from build123d import *

# Parameters (mm, degrees)
SKETCH1_R           = 5.85
SKETCH1_W           = 22.669
SKETCH1_H           = 11.7
BOSS_EXTRUDE1_DEPTH = 5.6


with BuildPart() as part:
    # Sketch1 → Boss-Extrude1 (new body)
    with BuildSketch(Plane.XY):
        Polygon((702.290264671, 402.743983564), (702.290264671, 391.585983564), (697.040264671, 391.585983564), (697.040264671, 387.985983564), (748.040264671, 387.985983564), (748.040264671, 393.985983564), (742.790264671, 393.985983564), (742.790264671, 400.343983564), (748.040264671, 400.343983564), (748.040264671, 406.343983564), (697.040264671, 406.343983564), (697.040264671, 402.743983564), align=None)
        with Locations((709.880764671, 397.164983564)):
            Circle(SKETCH1_R, mode=Mode.SUBTRACT)
        with Locations((728.805764671, 397.164983564)):
            Rectangle(SKETCH1_W, SKETCH1_H, mode=Mode.SUBTRACT)
    extrude(amount=BOSS_EXTRUDE1_DEPTH)


solid = part.part
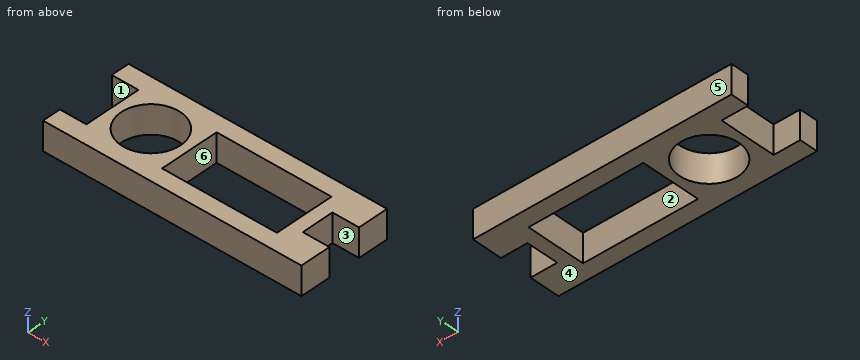
Read the model definition and answer for the solid it produces. Units are mm, in the model's axes. Face numbers are marked on the shaded views. A direction names the side the tool comes from. Round coordinates to 2 decimals unless told otherwise and drop trailing zeros. Write each loop counter-clockwise with the first axis right and the second up, starting at its lowest first coordinate (ties: lowest second). Pieces come first, ordered by that corner, then holes. Notation, with made-up numbers: (32, 49) - (51, 49) arc R23 ccw to (51, 73) - close; hole circle Ø8 at (-12, 9). An arc over 180 degrees is marked (long way). One line per question, with ' | ' between items. Start each with the question number.
1. Find the intervals of material crossed by probe 1 along Y at (x, z) = (726, 0.65); probe 2 along Y at (x, z) = (744, 1.9); probe 3 along X at (y, z) = (393, 4.15), in increasing order. Write a range as [from, to].
2. Section D-D (x = 701) is taken. Determine the outline of the cut face in (y, z), and give its area (3 significant figures).
3. This flat-tipped pin is pushed along its axis until it touches: pin 1 (1 mm diameter, centred on y = 395.5, z = 3, fed in from -X). Where does it stop, or does it pass through?
4. For the marked faces 1, 2 and 3, determine the directions among +Z, -Z, +X, -X, +Y, -Y from which every point of the face is accessible in a straight line to the end or side of a thin tool.
5. For a pull along Y with two mould halves and no side action, classify the marked faces 4, 5 and 6 as +Y half, -Y half, draft (parallel to the pull), parting line (faces both ways), or undercut.
6. Section C-C (z = 3.75) is taken. Determine the outline of the cut face in (x, y).
7. Section A-A (x = 723) is taken. Determine the outline of the cut face in (y, z).
8. Section B-B (y = 396) is taken. Determine the outline of the cut face in (x, z).
Filled in:
1) probe 1: [387.99, 391.31], [403.01, 406.34] | probe 2: [387.99, 393.99], [400.34, 406.34] | probe 3: [702.29, 705.77], [713.99, 717.47], [740.14, 748.04]
2) outline: (387.99, 0) - (391.59, 0) - (391.59, 5.6) - (387.99, 5.6) - close; (402.74, 0) - (406.34, 0) - (406.34, 5.6) - (402.74, 5.6) - close | area: 40.3 mm²
3) pin 1: x = 702.29
4) face 1: +Z, -Z, -X | face 2: +Z, -Z | face 3: +Z, -Z, +X
5) face 4: draft | face 5: +Y half | face 6: undercut
6) outline: (697.04, 387.99) - (748.04, 387.99) - (748.04, 393.99) - (742.79, 393.99) - (742.79, 400.34) - (748.04, 400.34) - (748.04, 406.34) - (697.04, 406.34) - (697.04, 402.74) - (702.29, 402.74) - (702.29, 391.59) - (697.04, 391.59) - close; hole circle Ø11.7 at (709.88, 397.16); hole (717.47, 391.31) - (740.14, 391.31) - (740.14, 403.01) - (717.47, 403.01) - close
7) outline: (387.99, 0) - (391.31, 0) - (391.31, 5.6) - (387.99, 5.6) - close; (403.01, 0) - (406.34, 0) - (406.34, 5.6) - (403.01, 5.6) - close
8) outline: (702.29, 0) - (704.15, 0) - (704.15, 5.6) - (702.29, 5.6) - close; (715.61, 0) - (717.47, 0) - (717.47, 5.6) - (715.61, 5.6) - close; (740.14, 0) - (742.79, 0) - (742.79, 5.6) - (740.14, 5.6) - close
